Autodesk Inventor part; units mm, degrees
ref_plane "YZ Plane" through (0, 0, 0) normal (1, 0, 0) x (0, 1, 0)
ref_plane "XZ Plane" through (0, 0, 0) normal (0, 1, 0) x (-1, 0, 0)
ref_plane "XY Plane" through (0, 0, 0) normal (0, 0, 1) x (1, 0, 0)
sketch "Náčrt2" plane through (0, 0, 0) normal (0, 0, 1) x (1, 0, 0)
  line L0 (-77, 0) -> (77, 0)
  line L1 (0, -77) -> (0, 77)
  line L2 (-55, 55) -> (55, 55)
  line L3 (55, 55) -> (55, -55)
  line L4 (55, -55) -> (-55, -55)
  line L5 (-55, -55) -> (-55, 55)
  point P0 (0, 0)
  dimension "d0" = 110
  dimension "d1" = 110
  dimension "d2" = 55
extrude "Vysunutí1" add sketch "Náčrt2" along normal blind 10
sketch "Náčrt3" plane through (0, 0, 10) normal (0, 0, 1) x (1, 0, 0)
  line L0 (-45, 45) -> (-7, 45)
  line L1 (-7, 45) -> (-7, 7)
  line L2 (-7, 7) -> (-45, 7)
  line L3 (-45, 7) -> (-45, 45)
  line L4 (-77, 0) -> (77, 0)
  line L5 (0, -77) -> (0, 77)
  line L6 (-55, 55) -> (-55, -55)
  line L7 (55, 55) -> (-55, 55)
  line L8 (7, 45) -> (45, 45)
  line L9 (7, 7) -> (7, 45)
  line L10 (45, 7) -> (7, 7)
  line L11 (45, 45) -> (45, 7)
  line L12 (-45, -7) -> (-7, -7)
  line L13 (-45, -45) -> (-45, -7)
  line L14 (-7, -45) -> (-45, -45)
  line L15 (-7, -7) -> (-7, -45)
  line L16 (7, -7) -> (45, -7)
  line L17 (7, -45) -> (7, -7)
  line L18 (45, -45) -> (7, -45)
  line L19 (45, -7) -> (45, -45)
  point P0 (0, 0)
  dimension "d5" = 38
  dimension "d6" = 38
  dimension "d7" = 10
  dimension "d8" = 10
  dimension "d11" = 52
  dimension "d14" = 52
extrude "Vysunutí2" cut sketch "Náčrt3" against normal blind 5 contours L0 L1 L2 L3 | L8 L11 L10 L9 | L12 L15 L14 L13 | L16 L19 L18 L17
fillet "Zaoblení1" radius 1 16 edges at (-45, 45, 7.5) (7, 45, 7.5) (-45, -7, 7.5) (7, -7, 7.5) (45, -45, 7.5) (-7, -45, 7.5) (45, 7, 7.5) (-7, 7, 7.5) (45, 45, 7.5) (-7, 45, 7.5) (45, -7, 7.5) (-7, -7, 7.5) (-45, -45, 7.5) (7, -45, 7.5) (7, 7, 7.5) (-45, 7, 7.5)
fillet "Zaoblení2" radius 4 4 edges at (-55, -55, 5) (55, -55, 5) (55, 55, 5) (-55, 55, 5)
equation "\"d1\" = d0"
equation "\"d2\" = 0.5 * d1"
equation "\"d6\" = d5"
equation "\"d8\" = d7"
equation "\"d14\" = d11"
properties part number "Paletka"
Model file for the job. Use its own axes, mm. A direction names the side the tool comes from. Give positions to 0.01 mm unless a question says otherwise; leave off trailing zeros. Write each loop counter-clockwise with the first axis right and the second up, starting at its lowest first coordinate (ties: lowest second). Pieces come first, ordered by that corner, then holes. Notation, with made-up numbers: (-13.5, 89) - (-2.5, 89) arc R31 cw to (-2.5, 118) - close; hole circle Ø7 at (-22, 20). An arc over 180 degrees is marked (long way). One line per question, with ' | ' between items. Start each with the question number.
(1) Slice it at A-A on y = -28. Write the cut outline in (x, z), plus the area to 3 significant figures.
(2) Slice it at C-C on z = 7.5. Give the number of separate pieces and of enclosed holes in the cut face, plus the area to 3 significant figures.
(3) Pin check, flat tip, straight feed: P1, Ø4, axis at x = -34, y = -33, coming from the +Z side. Stop position of the tip, or through.
(4) Wall check: line 1 along Y through (x, z) = (-42, 8.75); line 2 along Z through (x, y) = (-21, 33.5). Give the ranges that are in metal, low to high. Write a range as from..to.
(5) 3-axis set-ups, long thin cutter, end or side, ignore diameter. For faces 4 (the face through (1, -55, 5)), 5 (the face through (26, -45, 8)): which of +Z, -Z, +X, -X, +Y, -Y reach the whole face in a straight line?
(6) Two-plate mould, pull along X, no slides. Class faces 1 (the face through (53.797, -53.859, 5.07)), 2 (the face through (-53.859, -53.797, 5.07)), 3 (the face through (-26, -26, 5)): +X half, -X half, draft (parallel to the pull), parting line (faces both ways), or undercut.
Results below:
1) outline: (-55, 0) - (55, 0) - (55, 10) - (45, 10) - (45, 5) - (7, 5) - (7, 10) - (-7, 10) - (-7, 5) - (-45, 5) - (-45, 10) - (-55, 10) - close | area: 720 mm^2
2) separate pieces: 1 | enclosed holes: 4 | area: 6,310 mm^2
3) P1: z = 5
4) line 1: -55..-45, -7..7, 45..55 | line 2: 0..5
5) face 4: +Z, -Z, +X, -X, -Y | face 5: +Z
6) face 1: +X half | face 2: -X half | face 3: undercut
